```python
from build123d import *

# Parameters (mm, degrees)
F1_DEPTH = 25.4
F3_DEPTH = 2.54
F4_R     = 13.97
F5_DEPTH = 12.7


with BuildPart() as f1:
    # F0 (on Front) → F1 (new body)
    with BuildSketch(Plane.XZ):
        with BuildLine():
            ThreePointArc((51.606199, 22.347435), (49.735838, 24.639444), (46.905716, 25.500817))
            Line((46.905716, 25.500817), (-48.065889, 25.500817))
            ThreePointArc((-48.065889, 25.500817), (-57.046145, 21.781073), (-60.765889, 12.800817))
            Line((-60.765889, 12.800817), (-60.765889, -25.500817))
            Line((-60.765889, -25.500817), (-44.420032, -25.500817))
            ThreePointArc((-44.420032, -25.500817), (-38.1, -18.534626), (-31.779968, -25.500817))
            Line((-31.779968, -25.500817), (31.75, -25.500817))
            ThreePointArc((31.75, -25.500817), (38.1, -19.150817), (44.45, -25.500817))
            Line((44.45, -25.500817), (60.765889, -25.500817))
            Line((60.765889, -25.500817), (60.765889, -2.501722))
            ThreePointArc((60.765889, -2.501722), (60.526433, -0.047169), (59.817097, 2.314823))
            Line((59.817097, 2.314823), (51.606199, 22.347435))
        make_face()
    extrude(amount=F1_DEPTH)

    # F2 (on face) → F3 (cut)
    with BuildSketch(Plane.XZ.offset(25.4)):
        with BuildLine():
            Line((43.092143, 21.37755), (26.558064, 21.37755))
            ThreePointArc((26.558064, 21.37755), (24.762013, 20.633602), (24.018064, 18.83755))
            Line((24.018064, 18.83755), (24.018064, 8.465382))
            ThreePointArc((24.018064, 8.465382), (24.762013, 6.669331), (26.558064, 5.925382))
            Line((26.558064, 5.925382), (43.092143, 5.925382))
            ThreePointArc((43.092143, 5.925382), (44.888194, 6.669331), (45.632143, 8.465382))
            Line((45.632143, 8.465382), (45.632143, 18.83755))
            ThreePointArc((45.632143, 18.83755), (44.888194, 20.633602), (43.092143, 21.37755))
        make_face()
        with BuildLine():
            Line((20.232143, 8.465382), (20.232143, 18.83755))
            ThreePointArc((20.232143, 18.83755), (19.488194, 20.633602), (17.692143, 21.37755))
            Line((17.692143, 21.37755), (1.158064, 21.37755))
            ThreePointArc((1.158064, 21.37755), (-0.637987, 20.633602), (-1.381936, 18.83755))
            Line((-1.381936, 18.83755), (-1.381936, 8.465382))
            ThreePointArc((-1.381936, 8.465382), (-0.637987, 6.669331), (1.158064, 5.925382))
            Line((1.158064, 5.925382), (17.692143, 5.925382))
            ThreePointArc((17.692143, 5.925382), (19.488194, 6.669331), (20.232143, 8.465382))
        make_face()
        with BuildLine():
            Line((-5.167857, 8.465382), (-5.167857, 18.83755))
            ThreePointArc((-5.167857, 18.83755), (-5.911806, 20.633602), (-7.707857, 21.37755))
            Line((-7.707857, 21.37755), (-24.241936, 21.37755))
            ThreePointArc((-24.241936, 21.37755), (-26.037987, 20.633602), (-26.781936, 18.83755))
            Line((-26.781936, 18.83755), (-26.781936, 8.465382))
            ThreePointArc((-26.781936, 8.465382), (-26.037987, 6.669331), (-24.241936, 5.925382))
            Line((-24.241936, 5.925382), (-7.707857, 5.925382))
            ThreePointArc((-7.707857, 5.925382), (-5.911806, 6.669331), (-5.167857, 8.465382))
        make_face()
        with BuildLine():
            Line((-30.567857, 8.465382), (-30.567857, 18.83755))
            ThreePointArc((-30.567857, 18.83755), (-31.311806, 20.633602), (-33.107857, 21.37755))
            Line((-33.107857, 21.37755), (-49.641936, 21.37755))
            ThreePointArc((-49.641936, 21.37755), (-51.437987, 20.633602), (-52.181936, 18.83755))
            Line((-52.181936, 18.83755), (-52.181936, 8.465382))
            ThreePointArc((-52.181936, 8.465382), (-51.437987, 6.669331), (-49.641936, 5.925382))
            Line((-49.641936, 5.925382), (-33.107857, 5.925382))
            ThreePointArc((-33.107857, 5.925382), (-31.311806, 6.669331), (-30.567857, 8.465382))
        make_face()
    extrude(amount=-F3_DEPTH, mode=Mode.SUBTRACT)

    # F4 (on face) → F5 (cut)
    with BuildSketch(Plane.XZ.offset(25.4)):
        with Locations((-38.1, -24.884626)):
            Circle(F4_R)
        with Locations((38.1, -25.500817)):
            Circle(F4_R)
    extrude(amount=-F5_DEPTH, mode=Mode.SUBTRACT)

    # F6: F1 across plane


with BuildPart() as f1_1:
    add(f1.part)
    add(f1.part.mirror(Plane.XZ))


solid = f1_1.part
```
Build history of the part. All positions in model axes, mm. A direction names the side the tool comes from. Coordinates: 2 decimals unless noted, no trailing zeros. Order: outer loops, then holes, each group sorted by start corner. A loop starts at its lowest first (then second) coordinate and runs counter-clockwise, first axis right, second up.
Item 1: Saw through at B-B on y = -17. List the corners of the cut face in (x, z).
Filled in:
outline: (-60.77, -25.5) - (-52.06, -25.5) arc R13.97 cw (long way) to (-24.14, -25.5) - (24.13, -25.5) arc R13.97 cw to (52.07, -25.5) - (60.77, -25.5) - (60.77, -2.5) arc R12.7 ccw to (59.82, 2.31) - (51.61, 22.35) arc R5.08 ccw to (46.91, 25.5) - (-48.07, 25.5) arc R12.7 ccw to (-60.77, 12.8) - close
Item 2: Drill centre lines: L1, parallel to X at y = 16, z = -17.5; L2, parallel to Y at x = 9.5, z = 7; L3, parallel to X at y = 3, z = -21. Where is each one in solid material? Low to high.
Filled in:
L1: x = -60.77 to -49.96, -26.24 to 26.65, 49.55 to 60.77
L2: y = -22.86 to 22.86
L3: x = -60.77 to -43.12, -33.08 to 33.62, 42.58 to 60.77
Item 3: Tool access for faces 5 (the cylindrical face through (-26.02, 24.15, 20.65)), 6 (the cylindrical face through (-5.93, -24.15, 6.65)): list every direction of +Z, -Z, +X, -X, +Y, -Y with a clear straight run to the whole face (end or side of a thin tool).
Filled in:
face 5: +Y
face 6: -Y
Item 4: Mould opens along Z. For faces 1 (the cylindrical face through (24.74, 24.15, 6.69)), 2 (the cylindrical face through (-5.93, 24.15, 6.65)), 3 (the flat face through (-1, 25.4, 0)), 4 (the cylindrical face through (38.407, -19.139, -11.534)) say: released by +Z, released by -Z, zero draft, split by the parting line, or undercut.
Filled in:
face 1: undercut
face 2: undercut
face 3: zero draft
face 4: released by -Z
Item 5: Saw through at A-A on x = -38.1. List the corners of the cut face in (y, z), then the cut area to 3 significant figures.
Filled in:
outline: (-25.4, -10.91) - (-12.7, -10.91) - (-12.7, -18.53) - (12.7, -18.53) - (12.7, -10.91) - (25.4, -10.91) - (25.4, 5.93) - (22.86, 5.93) - (22.86, 21.38) - (25.4, 21.38) - (25.4, 25.5) - (-25.4, 25.5) - (-25.4, 21.38) - (-22.86, 21.38) - (-22.86, 5.93) - (-25.4, 5.93) - close
area: 1,960 mm2
Item 6: Saw through at C-C on x = 38.1. List the corners of the cut face in (y, z).
Filled in:
outline: (-25.4, -11.53) - (-12.7, -11.53) - (-12.7, -19.15) - (12.7, -19.15) - (12.7, -11.53) - (25.4, -11.53) - (25.4, 5.93) - (22.86, 5.93) - (22.86, 21.38) - (25.4, 21.38) - (25.4, 25.5) - (-25.4, 25.5) - (-25.4, 21.38) - (-22.86, 21.38) - (-22.86, 5.93) - (-25.4, 5.93) - close
Item 7: Drop flat-ended pins along their axis: pin 1 Ø1.5 at (y, z) = (-18.5, 2) entering from +X; pin 2 Ø7.5 at (x, z) = (-36, -17) entering from -Y; pin 3 Ø7.5 at (x, z) = (-46, 14.5) entering from -Y; pin 4 Ø17 at (x, z) = (32.5, 16.5) entering from +Y. Give the stop position or say it passes through.
Filled in:
pin 1: stops at x = 60.2
pin 2: stops at y = -12.7
pin 3: stops at y = -22.86
pin 4: stops at y = 25.4
